Here's how the part is built. I have some questions about the finished solid (model axes, mm). A direction names the side the tool comes from. Coordinates: 2 decimals unless noted, no trailing zeros. Loops run counter-clockwise (first coordinate to the right, second up) from the corner with the lowest first, then second, coordinate; pieces in that order, holes last. Notation, with made-up numbers: (62, 2.25) -> (72, 2.25) arc R24 cw to (72, 15.25) -> close; hole circle Ø11 at (39, -31). An arc over 180 degrees is marked (long way). Answer as a JSON object with one key per item and string values. Group by question number.
Q1. I need wall thicknesses on line 1 (X direction, y = 8.5, z = 0); line 2 (Y direction, x = -4.5, z = 4); line 3 (Z direction, x = 0, y = 4). Which ranges of each line are inside material? Lowest first, please.
Q2. I want a section at D-D on y = 17. Write out the boundary of the cut face in (x, z).
Q3. On a 3-axis mill with a long thin cutter (end or side, diameter ignored), from which of +Z, -Z, +X, -X, +Y, -Y can I reach the whole of each face in a straight line? I mean faces 1 (the cylindrical face through (6.03, 13.7, -2.47)), 2 (the flat face through (-5, 12.7, 5)), 3 (the flat face through (0, 12.7, 0)). Say none if no direction works.
Q4. I want a section at B-B on y = 10. Write out the boundary of the cut face in (x, z), then the cut area to 3 significant figures.
Q5. Thinking about a two-plate mould opening in X: for faces 4 (the conical face through (-0.84, 19.4, -2.67)), 5 (the cylindrical face through (1.99, 9.46, 5.25)), 6 (the cylindrical face through (0.2, 6.26, -4.48)), 7 (the flat face through (-6.515, 6, 0)), which applies, released by +X, released by -X, zero draft, split by the parting line, or undercut?
Q6. I want a section at C-C on y = 39. Write out the boundary of the cut face in (x, z), then the cut area to 3 significant figures.
Q7. I'm going to push flat-ended pins straight in: pin 1 (5 mm diameter, centred on x = 3.5, z = 3.5, fed in from +Y); pin 2 (1.5 mm diameter, centred on y = 13.5, z = 3, fed in from +X); pin 3 (3 mm diameter, centred on x = 4.5, z = 1.5, fed in from +Y); pin 4 (3.5 mm diameter, centred on x = 0, y = 8.84, fed in from +Z). Where does each tip first touch, or does it pass through?
Q8. I want a section at A-A on x = 0. Count the separate pieces of the cut face and the enclosed holes in it, then the cut area to 3 significant figures.
```python
from build123d import *

# Parameters (mm, degrees)
SKETCH4_W           = 13.0302
SKETCH4_H           = 12.976851724
SKETCH4_R           = 4.4831
BOSS_EXTRUDE3_DEPTH = 12.7
SKETCH5_R           = 2.0828
CUT_EXTRUDE4_DEPTH  = 15.24
SKETCH6_R           = 6.5151
BOSS_EXTRUDE4_DEPTH = 2.032
SKETCH7_R           = 2.286
BOSS_EXTRUDE6_DEPTH = 30.48
CHAMFER1_SIZE       = 3.20923319
CHAMFER1_SIZE2      = 5.558554938


with BuildPart() as part:
    # Sketch4 → Boss-Extrude3 (new body)
    with BuildSketch(Plane(origin=(0, 0, 0), x_dir=(1, 0, 0), z_dir=(0, 1, 0))):
        Rectangle(SKETCH4_W, SKETCH4_H)
        with Locations(Location((0, 0, 0), (0, 0, 270))):
            Circle(SKETCH4_R, mode=Mode.SUBTRACT)
    extrude(amount=BOSS_EXTRUDE3_DEPTH)

    # Sketch5 → Cut-Extrude4 (cut)
    with BuildSketch(Plane.XY.offset(6.488425862)):
        with Locations((0, 8.8392)):
            Circle(SKETCH5_R)
    extrude(amount=-CUT_EXTRUDE4_DEPTH, mode=Mode.SUBTRACT)

    # Sketch6 → Boss-Extrude4 (add)
    with BuildSketch(Plane(origin=(0, 12.7, 0), x_dir=(1, 0, 0), z_dir=(0, 1, 0))):
        with Locations(Location((0, 0, 0), (0, 0, 84.813545561))):
            Circle(SKETCH6_R)
    extrude(amount=BOSS_EXTRUDE4_DEPTH)

    # Sketch7 → Boss-Extrude6 (add)
    with BuildSketch(Plane(origin=(0, 14.732, 0), x_dir=(1, 0, 0), z_dir=(0, 1, 0))):
        with Locations(Location((0, 0, 0), (0, 0, 90))):
            Circle(SKETCH7_R)
    extrude(amount=BOSS_EXTRUDE6_DEPTH)

    # Chamfer1
    chamfer1_edges = [part.edges().sort_by_distance(p)[0] for p in [
        (0, 14.732, 2.286),
    ]]
    chamfer1_side = [part.faces().sort_by_distance(p)[0] for p in [
        (-0.572288462, 14.732, 6.304905465),
    ]]
    chamfer(chamfer1_edges, length=CHAMFER1_SIZE, length2=CHAMFER1_SIZE2, reference=chamfer1_side[0])


solid = part.part
```
Result set:
{
 "1": {"line 1": "x = -6.52 to -4.48, 4.48 to 6.52", "line 2": "y = 0 to 14.73", "line 3": "z = -6.49 to -4.48, 4.48 to 6.49"},
 "2": {"outline": "circle Ø8.37 at (0, 0)"},
 "3": {"face 1": "+Y", "face 2": "+Z, -X, +Y", "face 3": "-Y"},
 "4": {"outline": "(-6.52, -6.49) -> (-1.73, -6.49) -> (-1.73, -4.14) arc R4.48 cw to (-1.73, 4.14) -> (-1.73, 6.49) -> (-6.52, 6.49) -> close; (1.73, -6.49) -> (6.52, -6.49) -> (6.52, 6.49) -> (1.73, 6.49) -> (1.73, 4.14) arc R4.48 cw to (1.73, -4.14) -> close", "area": "91.3 mm²"},
 "5": {"face 4": "split by the parting line", "face 5": "undercut", "face 6": "undercut", "face 7": "released by -X"},
 "6": {"outline": "circle Ø4.57 at (0, 0)", "area": "16.4 mm²"},
 "7": {"pin 1": "stops at y = 20.01", "pin 2": "stops at x = 6.11", "pin 3": "stops at y = 18.63", "pin 4": "passes through"},
 "8": {"separate pieces": "3", "enclosed holes": "0", "area": "218 mm²"}
}
